Read the model definition and answer for the solid it produces. Units are mm, in the model's axes. Coordinates: 2 decimals unless noted, no trailing zeros. Order: outer loops, then holes, each group sorted by start corner. A loop starts at its lowest first (then second) coordinate and runs counter-clockwise, first axis right, second up. Notation, with made-up numbers: M -7.75,59 L -1.75,59 A18 ccw -1.75,81 Z; hole C 18.25,6 d7. An arc over 180 degrees is marked long. Use a Markdown table: item, result. Add a question column.
1) Find section C-C on z = -75.5. Write down the section's boundary in (x, y).
2) Find section A-A on y = 3.4. Write down the section's boundary in (x, z) (3 decimals).
3) Find section B-B on x = 92.5. Write down the section's boundary in (y, z) (3 decimals).
4) Find the intervals of material crossed by probe 1 along Z at (x, y) = (80, 3.7) (3 decimals); probe 2 along X at (y, z) = (2.2, -13.5) (3 decimals); probe 3 along Z at (x, y) = (158, 0.7) (3 decimals), in increasing order. Write a range as [from, to].
5) Each of these flat-tipped pins is pushed along its axis until it touches: pin 1 Ø1 at (y, z) = (1.5, -43) entering from -X (3 decimals); pin 2 Ø1.4 at (x, y) = (174.5, 3) entering from +Z (3 decimals); pin 3 Ø1.4 at (x, y) = (84, 3) entering from +Z; pin 4 Ø6 at (x, z) = (20, -81) entering from -Y. Where does it stop, or does it pass through?
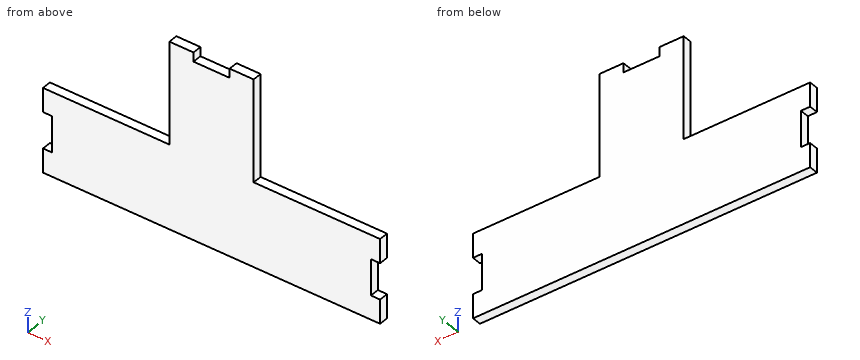
from build123d import *

# Parameters (mm, degrees)
SKETCH1_W           = 177.8
SKETCH1_H           = 98.425
BOSS_EXTRUDE1_DEPTH = 4.826
SKETCH2_W           = 4.826
SKETCH2_H           = 19.05
SKETCH2_W_2         = 19.05
SKETCH2_H_2         = 4.826
ALL_SLOTS_DEPTH     = 204.282096853
SKETCH3_W           = 66.675
SKETCH3_H           = 53.975
CUT_EXTRUDE2_DEPTH  = 204.282096853


with BuildPart() as part:
    # Sketch1 → Boss-Extrude1 (new body)
    with BuildSketch(Plane(origin=(0, 0, 0), x_dir=(1, 0, 0), z_dir=(0, 1, 0))):
        with Locations((88.9, 49.2125)):
            Rectangle(SKETCH1_W, SKETCH1_H)
    extrude(amount=BOSS_EXTRUDE1_DEPTH)

    # Sketch2 → All Slots (cut, through all)
    with BuildSketch(Plane(origin=(0, 4.826, 0), x_dir=(1, 0, 0), z_dir=(0, 1, 0))):
        with Locations((2.413, 76.2)):
            Rectangle(SKETCH2_W, SKETCH2_H)
        with Locations((175.387, 76.2)):
            Rectangle(SKETCH2_W, SKETCH2_H)
        with Locations((88.9, 2.413)):
            Rectangle(SKETCH2_W_2, SKETCH2_H_2)
    extrude(amount=-ALL_SLOTS_DEPTH, mode=Mode.SUBTRACT)

    # Sketch3 → Cut-Extrude2 (cut, through all)
    with BuildSketch(Plane(origin=(0, 4.826, 0), x_dir=(1, 0, 0), z_dir=(0, 1, 0))):
        with Locations((33.3375, 26.9875)):
            Rectangle(SKETCH3_W, SKETCH3_H)
        with Locations((144.4625, 26.9875)):
            Rectangle(SKETCH3_W, SKETCH3_H)
    extrude(amount=-CUT_EXTRUDE2_DEPTH, mode=Mode.SUBTRACT)


solid = part.part
Check result:
| question | item | result |
|---|---|---|
| 1 | outline | M 4.83,0 L 172.97,0 L 172.97,4.83 L 4.83,4.83 Z |
| 2 | outline | M 0,-98.425 L 177.8,-98.425 L 177.8,-85.725 L 172.974,-85.725 L 172.974,-66.675 L 177.8,-66.675 L 177.8,-53.975 L 111.125,-53.975 L 111.125,0 L 98.425,0 L 98.425,-4.826 L 79.375,-4.826 L 79.375,0 L 66.675,0 L 66.675,-53.975 L 0,-53.975 L 0,-66.675 L 4.826,-66.675 L 4.826,-85.725 L 0,-85.725 Z |
| 3 | outline | M 0,-98.425 L 4.826,-98.425 L 4.826,-4.826 L 0,-4.826 Z |
| 4 | probe 1 | z = [-98.425, -4.826] |
| 4 | probe 2 | x = [66.675, 111.125] |
| 4 | probe 3 | z = [-98.425, -53.975] |
| 5 | pin 1 | stops at x = 66.675 |
| 5 | pin 2 | stops at z = -53.975 |
| 5 | pin 3 | stops at z = -4.83 |
| 5 | pin 4 | stops at y = 0 |
